Check sheet for the modelled part. Datum: model origin and axes. Units: mm. A direction names the side the tool comes from. Give positions to 0.01 mm unless a question says otherwise; leave off trailing zeros. Order: outer loops, then holes, each group sorted by start corner. A loop starts at its lowest first (then second) coordinate and runs counter-clockwise, first axis right, second up. Notation, with made-up numbers: (23, 32) -> (76, 32) arc R14 ccw to (76, 50) -> close; hole circle Ø1 at (-28, 2.5). An arc over 180 degrees is marked (long way). One line per question, with ' | ' between items.
```python
from build123d import *

# Parameters (mm, degrees)
F1_DEPTH = 20
F3_DEPTH = 25
F4_W     = 25
F4_H     = 15
F5_DEPTH = 2


with BuildPart() as f1:
    # F0 (on Front) → F1 (new body)
    with BuildSketch(Plane.XZ):
        with BuildLine():
            ThreePointArc((3.5, 105), (0, 101.5), (-3.5, 105))
            Line((-3.5, 105), (-3.5, 110.5))
            ThreePointArc((-3.5, 110.5), (-4.37868, 112.62132), (-6.5, 113.5))
            Line((-6.5, 113.5), (-7, 113.5))
            ThreePointArc((-7, 113.5), (-9.12132, 112.62132), (-10, 110.5))
            Line((-10, 110.5), (-10, 25))
            ThreePointArc((-10, 25), (-12.928932, 17.928932), (-20, 15))
            Line((-20, 15), (-55, 15))
            ThreePointArc((-55, 15), (-58.535534, 13.535534), (-60, 10))
            Line((-60, 10), (-60, 0))
            Line((-60, 0), (-30, 0))
            Line((-30, 0), (-30, 1))
            ThreePointArc((-30, 1), (-29.414214, 2.414214), (-28, 3))
            Line((-28, 3), (28, 3))
            ThreePointArc((28, 3), (29.414214, 2.414214), (30, 1))
            Line((30, 1), (30, 0))
            Line((30, 0), (60, 0))
            Line((60, 0), (60, 10))
            ThreePointArc((60, 10), (58.535534, 13.535534), (55, 15))
            Line((55, 15), (20, 15))
            ThreePointArc((20, 15), (12.928932, 17.928932), (10, 25))
            Line((10, 25), (10, 110.5))
            ThreePointArc((10, 110.5), (9.12132, 112.62132), (7, 113.5))
            Line((7, 113.5), (6.5, 113.5))
            ThreePointArc((6.5, 113.5), (4.37868, 112.62132), (3.5, 110.5))
            Line((3.5, 110.5), (3.5, 105))
        make_face()
    extrude(amount=F1_DEPTH)

    # F2 (on face) → F3 (cut)
    with BuildSketch(Plane.YZ.offset(10)):
        Polygon((-4, 110.5), (-4, 116.603597), (-20, 116.603597), (-25.165081, 116.603597), (-25.165081, 79.442367), (-20, 79.442367), (-20, 81.5), (-20, 110.5), align=None)
        with BuildLine():
            Line((-4, 96.5), (-4, 110.5))
            Line((-4, 110.5), (-20, 110.5))
            Line((-20, 110.5), (-20, 81.5))
            ThreePointArc((-20, 81.5), (-17.949747, 86.449747), (-13, 88.5))
            Line((-13, 88.5), (-12, 88.5))
            ThreePointArc((-12, 88.5), (-6.343146, 90.843146), (-4, 96.5))
        make_face()
    extrude(amount=-F3_DEPTH, mode=Mode.SUBTRACT)

    # F4 (on face) → F5 (cut)
    with BuildSketch(Plane(origin=(0, 0, 0), x_dir=(1, 0, 0), z_dir=(0, 0, -1))):
        with Locations((-45, 10)):
            Rectangle(F4_W, F4_H)
        with Locations((45, 10)):
            Rectangle(F4_W, F4_H)
    extrude(amount=-F5_DEPTH, mode=Mode.SUBTRACT)


solid = f1.part
```
Q1. Section check C-C (z = 34). Enter the section's corners in (x, y), and give its area (3 significant figures).
Result sheet:
outline: (-10, -20) -> (10, -20) -> (10, 0) -> (-10, 0) -> close | area: 400 mm2
Q2. Mould release check, pull along X, two halves, no side actions. Record for faces 4 (the face through (60, -10, 5)), 5 (the face through (0, -20, 29)), 6 (the face through (0, -10, 3)): pulls with the +X half, pulls with the -X half, needs draft (parallel to the pull), parting line crosses it, or undercut.
Result sheet:
face 4: pulls with the +X half | face 5: needs draft | face 6: undercut
Q3. Section check A-A (x = -48). Enter the section's corners in (y, z).
Result sheet:
outline: (-20, 0) -> (-17.5, 0) -> (-17.5, 2) -> (-2.5, 2) -> (-2.5, 0) -> (0, 0) -> (0, 15) -> (-20, 15) -> close
Q4. Depth check by flat-ended pin: pin 1 Ø0.5 at (x, y) = (-2, -12.5) entering from +Z; pin 2 Ø12 at (x, y) = (-6, -7) entering from -Z; pin 3 Ø10 at (x, y) = (-41, -10.5) entering from +Z; pin 4 Ø1.6 at (x, z) = (46, 0.5) entering from +Y. Enter the tip coordinate at first touch or a pass-through.
Result sheet:
pin 1: stops at z = 88.5 | pin 2: stops at z = 3 | pin 3: stops at z = 15 | pin 4: stops at y = 0
Q5. Section check B-B (y = -7). Enter the section's corners in (x, z) (3 decimals), and give its area (3 significant figures).
Result sheet:
outline: (-60, 0) -> (-57.5, 0) -> (-57.5, 2) -> (-32.5, 2) -> (-32.5, 0) -> (-30, 0) -> (-30, 1) arc R2 cw to (-28, 3) -> (28, 3) arc R2 cw to (30, 1) -> (30, 0) -> (32.5, 0) -> (32.5, 2) -> (57.5, 2) -> (57.5, 0) -> (60, 0) -> (60, 10) arc R5 ccw to (55, 15) -> (20, 15) arc R10 cw to (10, 25) -> (10, 90.255) -> (-10, 90.255) -> (-10, 25) arc R10 cw to (-20, 15) -> (-55, 15) arc R5 ccw to (-60, 10) -> close | area: 3,060 mm2
Q6. Thickness scan on line 1 (X direction, y = -15, z = 84.5); line 2 (Z direction, x = 27.5, y = -7.75); line 3 (Y direction, x = -5, z = 98). Record the ranges inside material, lowest first.
Result sheet:
line 1: x = -10 to 10 | line 2: z = 3 to 15 | line 3: y = -4 to 0
Q7. Section check D-D (x = 0). Enter the section's corners in (y, z).
Result sheet:
outline: (-20, 3) -> (0, 3) -> (0, 101.5) -> (-4, 101.5) -> (-4, 96.5) arc R8 cw to (-12, 88.5) -> (-13, 88.5) arc R7 ccw to (-20, 81.5) -> close
Q8. Access from +Z, -Z, +X, -X, +Y, -Y to the whole of each face (thin tool, end or side, straight path). Record for faces 1 (the face through (-37, -10, 15)), 2 (the face through (10, -10, 58)), 3 (the face through (4.4, -1.97, 112.64)).
Result sheet:
face 1: +Z, -X, +Y, -Y | face 2: +Z, +X, +Y, -Y | face 3: +Z, +Y, -Y
